from build123d import *

# Parameters (mm, degrees)
F0_W     = 101.6
F0_H     = 76.2
F1_DEPTH = 38.1
F2_T     = -4.7625
F3_W     = 92.075
F3_H     = 66.675
F3_W_2   = 86.8494564931
F3_H_2   = 63.0672035732
F4_DEPTH = 31.75
F5_R     = 0.762
F6_R     = 5.08
F7_R     = 5.08


with BuildPart() as f1:
    # F0 (on Top) → F1 (new body)
    with BuildSketch(Plane.XY):
        Rectangle(F0_W, F0_H)
    extrude(amount=F1_DEPTH)

    # F2
    f2_openings = [f1.faces().sort_by_distance(p)[0] for p in [
        (0, 0, 38.1),
    ]]
    offset(amount=F2_T, openings=f2_openings)

    # F3 (on face) → F4 (join)
    with BuildSketch(Plane.XY.offset(4.7625)):
        Rectangle(F3_W, F3_H)
        Rectangle(F3_W_2, F3_H_2, mode=Mode.SUBTRACT)
    extrude(amount=F4_DEPTH)

    # F5
    f5_edges = [f1.edges().sort_by_distance(p)[0] for p in [
        (-46.0375, 33.3375, 37.30625),
        (46.0375, 33.3375, 37.30625),
        (46.0375, -33.3375, 37.30625),
        (-46.0375, -33.3375, 37.30625),
    ]]
    fillet(f5_edges, radius=F5_R)

    # F6
    f6_edges = [f1.edges().sort_by_distance(p)[0] for p in [
        (43.424728, 31.533602, 20.6375),
        (43.424728, -31.533602, 20.6375),
        (-43.424728, -31.533602, 20.6375),
        (-43.424728, 31.533602, 20.6375),
    ]]
    fillet(f6_edges, radius=F6_R)

    # F7
    f7_edges = [f1.edges().sort_by_distance(p)[0] for p in [
        (50.8, 38.1, 19.05),
        (50.8, -38.1, 19.05),
        (-50.8, 38.1, 19.05),
        (-50.8, -38.1, 19.05),
    ]]
    fillet(f7_edges, radius=F7_R)


solid = f1.part
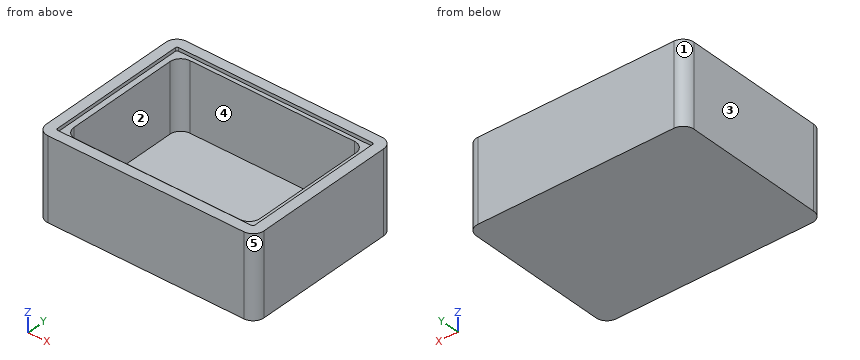
Input: part model. Units: mm. Frame: model coordinates. Face numbers are marked on the shaded views. A direction names the side the tool comes from. Coordinates: 2 decimals unless noted, no trailing zeros. Loops run counter-clockwise (first coordinate to the right, second up) from the corner with the lowest first, then second, coordinate; pieces in that order, holes last.
Q1. Cut plane B-B (y = -17.5). Output: boundary loops of the cut face in (x, z).
Q2. Cut plane A-A (z = 10). Output: boundary loops of the cut face in (x, y), then the cut area to 3 significant figures.
Q3. Contact query for a flat-ended pin moving along its axis: pin 1 (4 mm diameter, centred on x = -31, y = 17.5, fed in from +Z). Output: stop coordinate, or through.
Q4. Draft query along Y for the marked faces 3, 4 and 5. Return one class per face: +Y half, -Y half, draft (parallel to the pull), parting line (faces both ways), or undercut.
Q5. Cut plane C-C (x = -21). Output: boundary loops of the cut face in (y, z), then the cut area to 3 significant figures.
Q6. Set-up query: the marked faces 1 and 2. Return all of +Z, -Z, +X, -X, +Y, -Y with unobstructed straight access to the full face (end or side cutting, diameter ignored); none if empty.
Q7. Material intervals for line 1 (Y direction, x = 35.5, z = 32.5); line 2 (X direction, y = 23.5, z = 5); line 3 (Z direction, x = 33, y = 11), sorted ascending.
Working result:
1. outline: (-50.8, 0) - (50.8, 0) - (50.8, 38.1) - (46.04, 38.1) - (46.04, 36.51) - (43.42, 36.51) - (43.42, 4.76) - (-43.42, 4.76) - (-43.42, 36.51) - (-46.04, 36.51) - (-46.04, 38.1) - (-50.8, 38.1) - close
2. outline: (-50.8, -33.02) arc R5.08 ccw to (-45.72, -38.1) - (45.72, -38.1) arc R5.08 ccw to (50.8, -33.02) - (50.8, 33.02) arc R5.08 ccw to (45.72, 38.1) - (-45.72, 38.1) arc R5.08 ccw to (-50.8, 33.02) - close; hole (-43.42, -26.45) arc R5.08 ccw to (-38.34, -31.53) - (38.34, -31.53) arc R5.08 ccw to (43.42, -26.45) - (43.42, 26.45) arc R5.08 ccw to (38.34, 31.53) - (-38.34, 31.53) arc R5.08 ccw to (-43.42, 26.45) - close
2. area: 2,260 mm2
3. pin 1: stops at z = 4.76
4. face 3: draft
4. face 4: undercut
4. face 5: -Y half
5. outline: (-38.1, 0) - (38.1, 0) - (38.1, 38.1) - (33.34, 38.1) - (33.34, 36.51) - (31.53, 36.51) - (31.53, 4.76) - (-31.53, 4.76) - (-31.53, 36.51) - (-33.34, 36.51) - (-33.34, 38.1) - (-38.1, 38.1) - close
5. area: 795 mm2
6. face 1: +Z, -Z, -X, +Y
6. face 2: +Z
7. line 1: y = -38.1 to -31.53, 31.53 to 38.1
7. line 2: x = -50.8 to -43.42, 43.42 to 50.8
7. line 3: z = 0 to 4.76
